For this review, take the finished solid that the model builds, in its own axes (mm). A direction names the side the tool comes from. Give positions to 0.01 mm unless a question says otherwise; leave off trailing zeros. Write each loop counter-clockwise with the first axis right and the second up, starting at its lowest first coordinate (ties: lowest second). Pieces come first, ordered by that corner, then holes.
from build123d import *

# Parameters (mm, degrees)
CYLINDER058_R     = 1.75
CYLINDER058_DEPTH = 15
CYLINDER057_R     = 1.75
CYLINDER057_DEPTH = 15
EXTRUDE001_DEPTH  = 4


with BuildPart() as m3holds026:
    # Cylinder058 → Cylinder058 (new body)
    with BuildSketch(Plane(origin=(14.6, 0.25, 61.5), x_dir=(1, 0, 0), z_dir=(0, -1, 0))):
        Circle(CYLINDER058_R)
    extrude(amount=CYLINDER058_DEPTH)


with BuildPart() as fusion066:
    # Cylinder057 → Cylinder057 (new body)
    with BuildSketch(Plane(origin=(6, 0.25, 82), x_dir=(1, 0, 0), z_dir=(0, -1, 0))):
        Circle(CYLINDER057_R)
    extrude(amount=CYLINDER057_DEPTH)

    # Fusion066: union m3Holds026
    add(m3holds026.part)


with BuildPart() as c4holdtopleft:
    # Sketch003 → Extrude001 (new body)
    with BuildSketch(Plane.XZ):
        with BuildLine():
            Line((4.549471, 57.267887), (0.883944, 66.268614))
            Line((0.883944, 78.654398), (0.883944, 66.268614))
            ThreePointArc((6.613358, 86.871608), (2.353967, 83.73544), (0.883944, 78.654398))
            Line((6.613358, 85.92654), (6.613358, 86.871608))
            ThreePointArc((6.613358, 85.92654), (6.959213, 84.860057), (7.986391, 84.410718))
            Line((10.364112, 84.410718), (7.986391, 84.410718))
            Line((10.364112, 71.120834), (10.364112, 84.410718))
            Line((17.859817, 64.935078), (10.364112, 71.120834))
            ThreePointArc((15.746783, 57.267887), (19.454521, 60.370821), (17.859817, 64.935078))
            Line((4.549471, 57.267887), (15.746783, 57.267887))
        make_face()
    extrude(amount=EXTRUDE001_DEPTH)


with BuildPart() as c4holdtopleft_1:
    # Extrude001 placement: moved
    add(c4holdtopleft.part.moved(Location((0, -8, 0))))

    # Cut011: cut Fusion066
    add(fusion066.part, mode=Mode.SUBTRACT)


solid = c4holdtopleft_1.part
(1) We need section A-A (y = -10.2). Write out the cut boundary in (x, z).
(2) Tool access review of faces 5 (the cylindrical face through (19.435, -9.972, 60.302)), 6 (the flat face through (6.613, -10, 86.4)): name each direction out of +Z, -Z, +X, -X, +Y, -Y from which nothing blocks a thin tool from reaching the whole face with its end or side.
(3) For L1, parallel to X at y = -11.4, z = 78.5; L2, parallel to X at y = -10.2, z = 82; L3, parallel to Z at x = 14.6, y = -10, list the stretches that pass through material, from the lowest coordinate up.
(4) We need section D-D (z = 76.5). Write out the cut boundary in (x, y), and give its area (3 significant figures).
(5) We need section B-B (z = 61.5). Write out the cut boundary in (x, y).
(6) The part is to be moulded in two halves that separate along X. For faces 1 (the flat face through (8, -12, 69)), 2 (the flat face through (10.364, -10, 78)), 3 (the cylindrical face through (15.41, -9.97, 59.95)), 4 (the cylindrical face through (2.4, -10, 83.8)), say which applies: +X half, -X half, draft (parallel to the pull), parting line (faces both ways), or undercut.
(7) We need section C-C (x = 14.6). Write out the cut boundary in (y, z).
(8) Clearance check with flat-ended pins moving along their axes: pin 1 Ø2 at (y, z) = (-9.5, 76.5) entering from +X; pin 2 Ø1.2 at (y, z) = (-11, 71) entering from -X; pin 3 Ø0.7 at (x, y) = (9.5, -11) entering from +Z. State where each tip first meets the part, or that it passes through.
The answers:
1. outline: (0.88, 66.27) - (4.55, 57.27) - (15.75, 57.27) arc R4.25 ccw to (17.86, 64.94) - (10.36, 71.12) - (10.36, 84.41) - (7.99, 84.41) arc R1.37 cw to (6.61, 85.93) - (6.61, 86.87) arc R8.23 ccw to (0.88, 78.65) - close; hole circle Ø3.5 at (6, 82); hole circle Ø3.5 at (14.6, 61.5)
2. face 5: +X, +Y, -Y
2. face 6: +Z, +X, +Y, -Y
3. L1: x = 0.88 to 10.36
3. L2: x = 1.43 to 4.25, 7.75 to 10.36
3. L3: z = 57.27 to 59.75, 63.25 to 67.63
4. outline: (0.88, -12) - (10.36, -12) - (10.36, -8) - (0.88, -8) - close
4. area: 37.9 mm2
5. outline: (2.83, -12) - (12.85, -12) - (12.85, -8) - (2.83, -8) - close; (16.35, -12) - (19.61, -12) - (19.61, -8) - (16.35, -8) - close
6. face 1: draft
6. face 2: +X half
6. face 3: undercut
6. face 4: -X half
7. outline: (-12, 57.27) - (-8, 57.27) - (-8, 59.75) - (-12, 59.75) - close; (-12, 63.25) - (-8, 63.25) - (-8, 67.63) - (-12, 67.63) - close
8. pin 1: stops at x = 10.36
8. pin 2: stops at x = 0.88
8. pin 3: stops at z = 84.41
